The drawing under review shows one solid part. Ordinate dimensions are in mm from its lowest x, y, z. A direction names the side the tool comes from. Coordinates: 2 decimals unless noted, no trailing zeros. Write each loop counter-clockwise with the first axis right and the second up, starting at its lowest first coordinate (ties: lowest second). Pieces come first, ordered by that corner, then holes. Notation, with made-up numbers: (78.25, 73.25) -> (137.25, 73.25) arc R30 ccw to (137.25, 110.25) -> close; hole circle Ø2 at (87.5, 33). An arc over 180 degrees is marked (long way). Put each result on its own line as item: value. Start each with the question number.
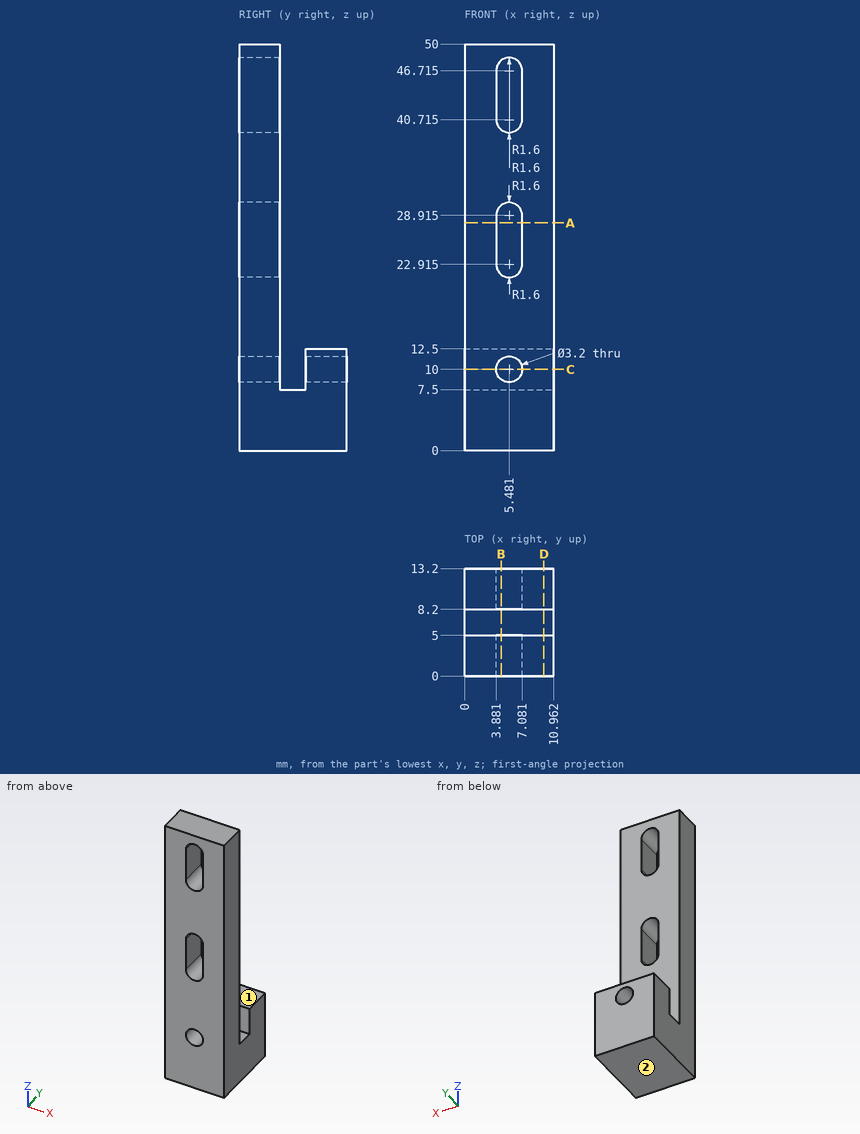
1. Consider section C-C on z = 10. State the section outline as (x, y) points.
2. Wall thickness on line 1 (X direction, y = 1.7, z = 10); line 2 (Y direction, x = 9, z = 8); line 3 (Z direction, x = 1, y = 6): over which ranges is each line inside the solid? List them lowest first. Write a range as from..to.
3. Insertion check: P1, Ø1.5, axis at y = 1.5, z = 25, coming from the -X side; P2, Ø6, axis at x = 4.5, y = 9.5, coming from the +Z side; P3, Ø1, axis at x = 8, z = 32.5, coming from the +Y side; P4, Ø2.5, axis at x = 5.48, z = 10, coming from the -Y side. Each pin has a flat end and moves straight along its axis. Give the tip position at first contact, or say it passes through.
4. Consider section A-A on z = 28. State the section outline as (x, y) points.
5. Tool access review of the marked faces 1 and 2: name each direction out of +Z, -Z, +X, -X, +Y, -Y from which nothing blocks a thin tool from reaching the whole face with its end or side.
6. Consider section B-B on x = 4.5. State the section outline as (y, z) points, then the cut area to 3 significant figures.
7. Consider section D-D on x = 9.75. State the section outline as (y, z) points.
Output values:
1. outline: (0, 0) -> (3.88, 0) -> (3.88, 5) -> (0, 5) -> close; (0, 8.2) -> (3.88, 8.2) -> (3.88, 13.2) -> (0, 13.2) -> close; (7.08, 0) -> (10.96, 0) -> (10.96, 5) -> (7.08, 5) -> close; (7.08, 8.2) -> (10.96, 8.2) -> (10.96, 13.2) -> (7.08, 13.2) -> close
2. line 1: x = 0..3.88, 7.08..10.96
2. line 2: y = 0..5, 8.2..13.2
2. line 3: z = 0..7.5
3. P1: stops at x = 0
3. P2: stops at z = 12.5
3. P3: stops at y = 5
3. P4: passes through
4. outline: (0, 0) -> (3.88, 0) -> (3.88, 5) -> (0, 5) -> close; (7.08, 0) -> (10.96, 0) -> (10.96, 5) -> (7.08, 5) -> close
5. face 1: +Z, +X, -X, +Y
5. face 2: -Z, +X, -X, +Y, -Y
6. outline: (0, 0) -> (13.2, 0) -> (13.2, 8.74) -> (8.2, 8.74) -> (8.2, 7.5) -> (5, 7.5) -> (5, 8.74) -> (0, 8.74) -> close; (0, 11.26) -> (5, 11.26) -> (5, 21.65) -> (0, 21.65) -> close; (0, 30.18) -> (5, 30.18) -> (5, 39.45) -> (0, 39.45) -> close; (0, 47.98) -> (5, 47.98) -> (5, 50) -> (0, 50) -> close; (8.2, 11.26) -> (13.2, 11.26) -> (13.2, 12.5) -> (8.2, 12.5) -> close
6. area: 226 mm^2
7. outline: (0, 0) -> (13.2, 0) -> (13.2, 12.5) -> (8.2, 12.5) -> (8.2, 7.5) -> (5, 7.5) -> (5, 50) -> (0, 50) -> close
